Work out the finished part from the listing and answer in its coordinate system (mm). A direction names the side the tool comes from. Give positions to 0.01 mm unless a question says otherwise; leave off trailing zeros. Order: outer loops, then holes, each group sorted by start corner. A loop starts at its lowest first (then second) coordinate and runs counter-clockwise, first axis right, second up. Notation, with made-up numbers: (46, 69) - (91, 69) arc R15 cw to (91, 75) - close; hole circle Ø9 at (-11, 62). An arc over 180 degrees is marked (long way). Write each question's results on one line, items separated by ' | '.
from build123d import *

# Parameters (mm, degrees)
F0_W     = 1190
F0_H     = 500
F1_DEPTH = 5
F2_W     = 500
F2_H     = 5
F2_H_2   = 2300
F3_DEPTH = 5


# Not quite as in the source:
# - the program builds the solid bodies; features that only make, move or delete a surface that nothing else refers to are left out


with BuildPart() as f1:
    # F0 (on Top) → F1 (new body)
    with BuildSketch(Plane.XY):
        Rectangle(F0_W, F0_H)
    extrude(amount=-F1_DEPTH)

    # F2 (on face) → F3 (join)
    with BuildSketch(Plane(origin=(-595, 0, 0), x_dir=(0, -1, 0), z_dir=(-1, 0, 0))):
        with Locations((0, -2.5)):
            Rectangle(F2_W, F2_H)
        with Locations((0, 1150)):
            Rectangle(F2_W, F2_H_2)
    extrude(amount=F3_DEPTH)


solid = f1.part
1. Straight lines are drawn through the part: line 1 (Z direction, x = -339.5, y = -112); line 2 (X direction, y = 168, z = 310.5). For each, find the intervals that lie inside material, in ascending order. Write a range as [from, to].
Answer list:
line 1: [-5, 0] | line 2: [-600, -595]
2. A cutting plane is placed at A-A, the plane y = -65. Write down the section's boundary in (x, z).
Answer list:
outline: (-600, -5) - (595, -5) - (595, 0) - (-595, 0) - (-595, 2300) - (-600, 2300) - close
3. A cutting plane is placed at B-B, the plane z = 1312. Write down the section's boundary in (x, y), then the cut area to 3 significant figures.
Answer list:
outline: (-600, -250) - (-595, -250) - (-595, 250) - (-600, 250) - close | area: 2,500 mm^2
4. A cutting plane is placed at C-C, the plane x = 146. Write down the section's boundary in (y, z).
Answer list:
outline: (-250, -5) - (250, -5) - (250, 0) - (-250, 0) - close
5. A tool of negligible diameter and unlimited length cuts with its end or side. For faces 1 (the face through (-8, 4, 0)), 2 (the face through (6, 3, -5)), from which of +Z, -Z, +X, -X, +Y, -Y can it reach the whole face along a straight path? Write none if from no direction.
Answer list:
face 1: +Z, +X, +Y, -Y | face 2: -Z, +X, -X, +Y, -Y
